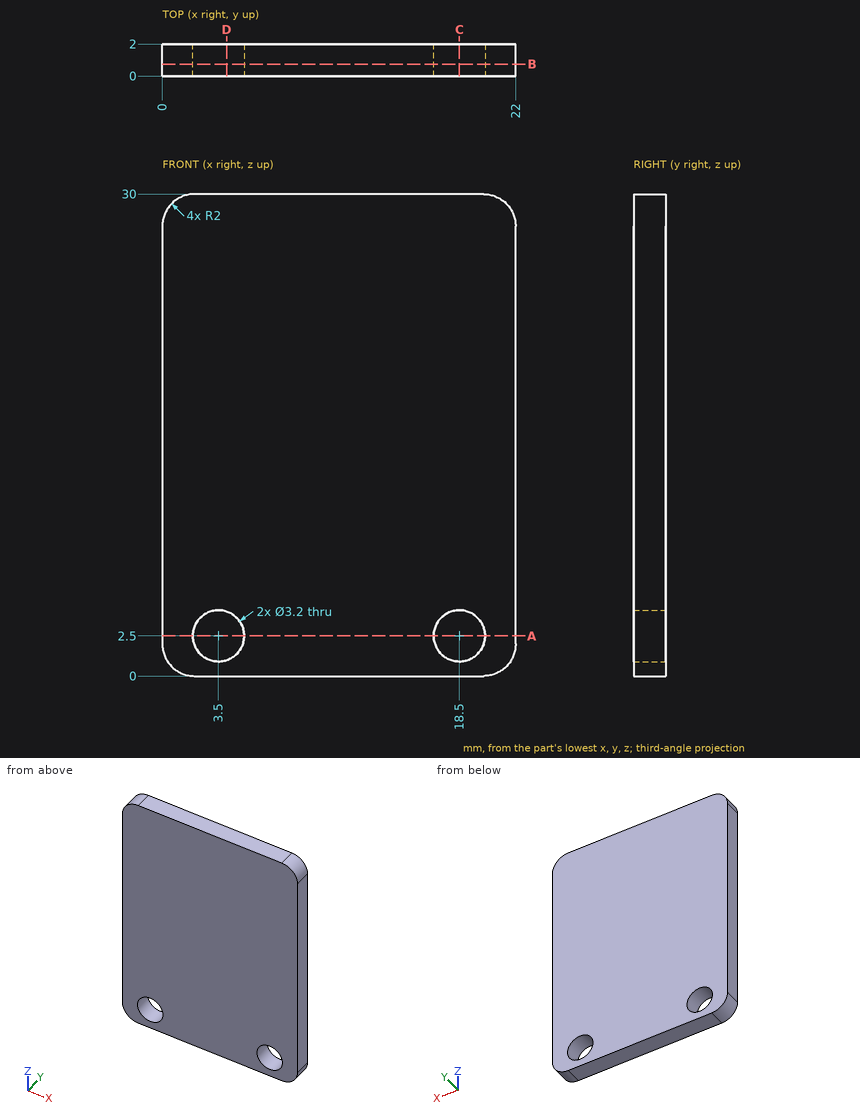
Could you check a few things on this drawing? It's one solid part, dimensions in mm from its lowest x, y, z. Coordinates: 2 decimals unless noted, no trailing zeros. Order: outer loops, then holes, each group sorted by start corner. A loop starts at its lowest first (then second) coordinate and runs counter-clockwise, first axis right, second up. Notation, with made-up numbers: M 51,27.5 L 75,27.5 A22 ccw 75,39.5 Z; hole C 76.25,21 d5. An arc over 180 degrees is marked long. Use one line per item in the form item = value. Start each with the question number.
1. Suppose I cut it at C-C on x = 18.5. Write out the boundary of the cut face in (y, z).
2. Please list where these lines run through material, in increasing order: line 1 (X direction, y = 1.3, z = 2.5); line 2 (Z direction, x = 18.5, y = 1.1); line 3 (Z direction, x = 17.25, y = 1).
3. Suppose I cut it at B-B on y = 0.75. Write out the boundary of the cut face in (x, z), then the cut area to 3 significant figures.
4. For pin 1 (3 mm diameter, centred on x = 3.5, z = 2.5, fed in from +Y), with a flat end and sliding along its axis, tell me the tip position at first contact or that it passes through.
5. Suppose I cut it at D-D on x = 4. Write out the boundary of the cut face in (y, z), then the cut area to 3 significant figures.
6. Suppose I cut it at A-A on z = 2.5. Write out the boundary of the cut face in (x, y).
Geometry says:
q1.outline = M 0,0 L 2,0 L 2,0.9 L 0,0.9 Z; M 0,4.1 L 2,4.1 L 2,30 L 0,30 Z
q2.line_1 = 0 to 1.9, 5.1 to 16.9, 20.1 to 22
q2.line_2 = 0 to 0.9, 4.1 to 30
q2.line_3 = 0 to 1.5, 3.5 to 30
q3.outline = M 0,2 A2 ccw 2,0 L 20,0 A2 ccw 22,2 L 22,28 A2 ccw 20,30 L 2,30 A2 ccw 0,28 Z; hole C 3.5,2.5 d3.2; hole C 18.5,2.5 d3.2
q3.area = 640 mm^2
q4.pin_1 = through
q5.outline = M 0,0 L 2,0 L 2,0.98 L 0,0.98 Z; M 0,4.02 L 2,4.02 L 2,30 L 0,30 Z
q5.area = 53.9 mm^2
q6.outline = M 0,0 L 1.9,0 L 1.9,2 L 0,2 Z; M 5.1,0 L 16.9,0 L 16.9,2 L 5.1,2 Z; M 20.1,0 L 22,0 L 22,2 L 20.1,2 Z
